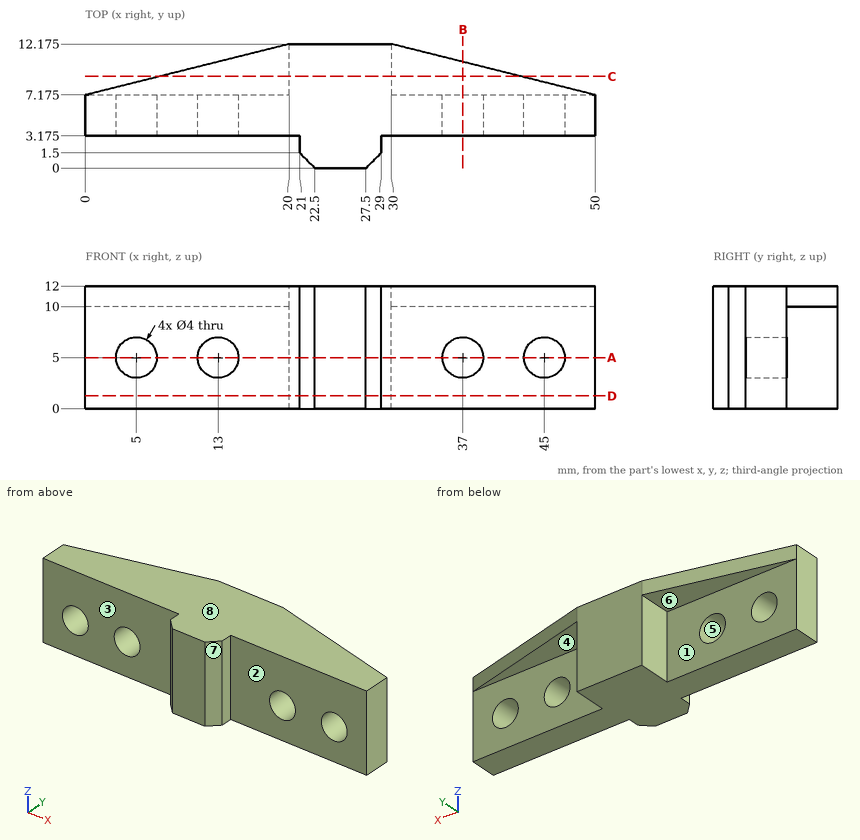
Geometry check sheet. Reference: drawing and pictorial views, mm from the part's lowest x, y, z. A direction names the side the tool comes from. Coordinates: 2 decimals unless noted, no trailing zeros. Order: outer loops, then holes, each group sorted by start corner. A loop starts at its lowest first (then second) coordinate and runs counter-clockwise, first axis right, second up.
Item 1: Tool access check on the marked faces 1, 2, 3 and 4. Record the directions out of +Z, -Z, +X, -X, +Y, -Y that give a thin tool (end or side, any length) a straight path to the whole face; none if there is none.
Item 2: Scan lines: line 1 along X through (y, z) = (4.05, 5); line 2 along Z through (x, y) = (13, 5.55); line 3 along Y through (x, z) = (37.5, 9.75) (3 decimals). Record each from-to range of solid material in increasing order.
Item 3: Section check D-D (z = 1.25). Enter the section's corners in (x, y) (3 decimals).
Item 4: Depth check by flat-ended pin: pin 1 (5 mm diameter, centred on x = 45, z = 5, fed in from +Y) (3 decimals); pin 2 (5 mm diameter, centred on y = 5.5, z = 3.5, fed in from -X); pin 3 (6 mm diameter, centred on x = 8, z = 8, fed in from -Y) (3 decimals); pin 4 (1.5 mm diameter, centred on x = 7.5, y = 10, fed in from -Z). Enter the tip coordinate at first touch or a pass-through.
Item 5: Section check B-B (x = 37). Enter the section's corners in (y, z) (3 decimals).
Item 6: Mould release check, pull along Z, two halves, no side actions. Record for the marked faces 5, 6, 7 and 8: released by +Z, released by -Z, zero draft, split by the parting line, or undercut.
Item 7: Section check A-A (z = 5). Count the separate pieces of the cut face and the enclosed holes in it, plus the area to 3 significant figures.
Item 8: Section check C-C (y = 9). Enter the section's corners in (x, z).
Check sheet entries:
1. face 1: -Z, -X, +Y
1. face 2: +Z, -Z, +X, -Y
1. face 3: +Z, -Z, -X, -Y
1. face 4: -Z, +X, +Y
2. line 1: x = 0 to 3, 7 to 11, 15 to 35, 39 to 43, 47 to 50
2. line 2: z = 0 to 3, 7 to 12
2. line 3: y = 3.175 to 7.175
3. outline: (0, 3.175) - (21, 3.175) - (21, 1.5) - (22.5, 0) - (27.5, 0) - (29, 1.5) - (29, 3.175) - (50, 3.175) - (50, 7.175) - (30, 7.175) - (30, 12.175) - (20, 12.175) - (20, 7.175) - (0, 7.175) - close
4. pin 1: stops at y = 7.175
4. pin 2: stops at x = 0
4. pin 3: stops at y = 3.175
4. pin 4: passes through
5. outline: (3.175, 0) - (7.175, 0) - (7.175, 3) - (3.175, 3) - close; (3.175, 7) - (7.175, 7) - (7.175, 10) - (10.425, 10) - (10.425, 12) - (3.175, 12) - close
6. face 5: undercut
6. face 6: released by -Z
6. face 7: zero draft
6. face 8: released by +Z
7. separate pieces: 5
7. enclosed holes: 0
7. area: 209 mm2
8. outline: (7.3, 10) - (20, 10) - (20, 0) - (30, 0) - (30, 10) - (42.7, 10) - (42.7, 12) - (7.3, 12) - close
